Autodesk Fusion 360 part; units mm, degrees
sketch "Sketch1" plane through (0, 0, 0) normal (0, 1, 0) x (1, 0, 0)
  circle A0 centre (-14.1, 0) radius 1.6
  circle A1 centre (14.1, 0) radius 1.6
  line L0 (17.6, 1.5) -> (17.6, -11.5)
  line L1 (12.6, -16.5) -> (-12.6, -16.5)
  line L2 (-17.6, -11.5) -> (-17.6, 1.5)
  line L3 (10.6, 1.5) -> (10.6, -7.5)
  line L4 (-10.6, -7.5) -> (-10.6, 1.5)
  line L5 (12.6, 3.5) -> (15.6, 3.5)
  line L6 (-15.6, 3.5) -> (-12.6, 3.5)
  arc A2 (-17.6, -11.5) -> (-12.6, -16.5) centre (-12.6, -11.5) ccw
  arc A3 (12.6, -16.5) -> (17.6, -11.5) centre (12.6, -11.5) ccw
  arc A4 (-15.6, 3.5) -> (-17.6, 1.5) centre (-15.6, 1.5) ccw
  arc A5 (-10.6, 1.5) -> (-12.6, 3.5) centre (-12.6, 1.5) ccw
  arc A6 (12.6, 3.5) -> (10.6, 1.5) centre (12.6, 1.5) ccw
  arc A7 (17.6, 1.5) -> (15.6, 3.5) centre (15.6, 1.5) ccw
  line L7 (10.6, -7.5) -> (10.6, -9.5)
  line L8 (10.6, -9.5) -> (-10.6, -9.5)
  line L9 (-10.6, -9.5) -> (-10.6, -7.5)
  dimension "d2" = 14.1
  dimension "d3" = 3.2
  dimension "d4" = 3.2
  dimension "d11" = 5
  dimension "d12" = 2
extrude "Extrude1" add sketch "Sketch1" along normal blind 7.5
sketch "Sketch2" plane through (0, 0, 9.5) normal (0, 0, -1) x (1, 0, 0)
  line L0 (8.6, 0) -> (-8.6, 0)
  line L1 (-12.6, 0) -> (12.6, 0)
  line L2 (-8, 0) -> (-2.6967, 0) construction
  line L3 (-12.6, 0) -> (12.6, 0)
  line L4 (10.6, 0) -> (-10.6, 0)
  line L5 (-10.6, 0) -> (-10.6, -7.5)
  line L6 (-10.6, -7.5) -> (10.6, -7.5)
  line L7 (10.6, -7.5) -> (10.6, 0)
  circle A0 centre (8, -3.75) radius 1.6
  line L8 (-12.6, -7.5) -> (-12.6, 0)
  line L9 (8, 0) -> (4.25, -3.75)
  line L10 (12.6, -7.5) -> (-12.6, -7.5)
  line L11 (0, -3.75) -> (8, -3.75)
  circle A1 centre (-8, -3.75) radius 1.6
  line L12 (12.6, 0) -> (12.6, -7.5)
  line L13 (-8, 0) -> (-4.25, -3.75)
  line L14 (0, -3.75) -> (-8, -3.75)
  point P0 (0, -3.75)
extrude "Extrude2" cut sketch "Sketch2" against normal blind 8 contours A0 | A1 | L0 L1 L3 L4 L9 L11 L13 L14
fillet "Fillet2" radius 1 4 edges at (-8, 0, 13) (-4.25, 3.75, 13) (4.25, 3.75, 13) (8, 0, 13)
chamfer "Chamfer5" distance 0.5 angle 45 44 edges at (-10.6, 7.5, 4) (-11.1858, 7.5, -2.9142) (-14.1, 7.5, -3.5) (-17.0142, 7.5, -2.9142) (-17.6, 7.5, 5) (-16.1355, 7.5, 15.0355) (0, 7.5, 16.5) (16.1355, 7.5, 15.0355) (17.6, 7.5, 5) (17.0142, 7.5, -2.9142) (14.1, 7.5, -3.5) (11.1858, 7.5, -2.9142) (10.6, 7.5, 4) (0, 7.5, 9.5) (-10.6, 0, 4) (-11.1858, 0, -2.9142) (-14.1, 0, -3.5) (-17.0142, 0, -2.9142) (-17.6, 0, 5) (-16.1355, 0, 15.0355) (-10.5071, 0, 16.5) (-8.0315, 0.0761, 16.5) (-6.125, 1.875, 16.5) (-4.2185, 3.6739, 16.5) (0, 3.75, 16.5) (4.2185, 3.6739, 16.5) (6.125, 1.875, 16.5) (8.0315, 0.0761, 16.5) (10.5071, 0, 16.5) (16.1355, 0, 15.0355) (17.6, 0, 5) (17.0142, 0, -2.9142) (14.1, 0, -3.5) (11.1858, 0, -2.9142) (10.6, 0, 4) (9.5071, 0, 9.5) (8.0315, 0.0761, 9.5) (6.125, 1.875, 9.5) (4.2185, 3.6739, 9.5) (0, 3.75, 9.5) (-4.2185, 3.6739, 9.5) (-6.125, 1.875, 9.5) (-8.0315, 0.0761, 9.5) (-9.5071, 0, 9.5)
Can you work these out from the model? Positions are in its coordinate system, mm. A direction names the side the tool comes from. Give positions to 0.01 mm unless a question says otherwise; leave off trailing zeros. Order: outer loops, then holes, each group sorted by start corner. A loop starts at its lowest first (then second) coordinate and runs counter-clockwise, first axis right, second up. Notation, with made-up numbers: (-25, 72) - (20, 72) arc R35 cw to (20, 110) - close; hole circle Ø4 at (40, 41.5). An arc over 180 degrees is marked (long way). Use a Markdown table: item, result. Add a question column.
Q1. Please list where these lines run through material, in increasing order: line 1 along X through (y, z) = (5.5, 6.75); line 2 along X through (y, z) = (4.75, 13.5); line 3 along X through (y, z) = (7, 0.5).
Q2. If we section it at B-B on z = 0: Write out the boundary of the cut face in (x, y), plus the area to 3 significant figures.
Q3. On a 3-axis mill with a long thin cutter (end or side, diameter ignored), from which of +Z, -Z, +X, -X, +Y, -Y can I reach the whole of each face in a straight line? I mean faces 4 (the flat face through (-6.282, 2.076, 9.746)), 5 (the flat face through (0, 3.75, 13)), 6 (the flat face through (-10.6, 4, 4)), 7 (the conical face through (11.43, 7.36, -2.65)). Say none if no direction works.
Q4. I'm going to push flat-ended pins straight in: pin 1 (3.5 mm diameter, centred on x = 8, y = 3.75, fed in from +Z); pin 2 (3 mm diameter, centred on x = 4.5, y = 3, fed in from -Z); pin 3 (6.5 mm diameter, centred on x = 1.5, z = 14, fed in from -Y); pin 4 (4 mm diameter, centred on x = 9, y = 2.5, fed in from -Z). Where does each tip first touch, or does it pass through?
Q5. If we section it at C-C on y = 2.5: Count the separate pieces of the cut face and the enclosed holes in it, plus the area to 3 significant figures.
Q6. If we mould it in two halves opening along Z, with no side actions, what happens to faces 1 (the flat face through (6.282, 2.076, 9.746)), 2 (the flat face through (17.6, 4, 5)), 3 (the cylindrical face through (-12.574, 3.698, 0.481))? For each: released by +Z, released by -Z, zero draft, split by the parting line, or undercut.
Q7. If we section it at A-A on y = 1: Write out the boundary of the cut face in (x, z).
Q8. If we section it at D-D on z = 2.75: Write out the boundary of the cut face in (x, y), plus the area to 3 significant figures.
Answers follow:
| question | item | result |
|---|---|---|
| 1 | line 1 | x = -17.6 to -10.6, 10.6 to 17.6 |
| 1 | line 2 | x = -17.18 to -9.25, -6.75 to 6.75, 9.25 to 17.18 |
| 1 | line 3 | x = -17.6 to -15.62, -12.58 to -10.6, 10.6 to 12.58, 15.62 to 17.6 |
| 2 | outline | (-17.6, 0.5) - (-17.1, 0) - (-15.7, 0) - (-15.7, 7.5) - (-17.1, 7.5) - (-17.6, 7) - close; (-12.5, 0) - (-11.1, 0) - (-10.6, 0.5) - (-10.6, 7) - (-11.1, 7.5) - (-12.5, 7.5) - close; (10.6, 0.5) - (11.1, 0) - (12.5, 0) - (12.5, 7.5) - (11.1, 7.5) - (10.6, 7) - close; (15.7, 0) - (17.1, 0) - (17.6, 0.5) - (17.6, 7) - (17.1, 7.5) - (15.7, 7.5) - close |
| 2 | area | 56.0 mm^2 |
| 3 | face 4 | -Z, -Y |
| 3 | face 5 | +Z, -Z, -Y |
| 3 | face 6 | -Z, +Y, -Y |
| 3 | face 7 | -Z, +Y |
| 4 | pin 1 | stops at z = 16.5 |
| 4 | pin 2 | stops at z = 9.5 |
| 4 | pin 3 | stops at y = 3.25 |
| 4 | pin 4 | stops at z = -2.7 |
| 5 | separate pieces | 4 |
| 5 | enclosed holes | 2 |
| 5 | area | 292 mm^2 |
| 6 | face 1 | released by -Z |
| 6 | face 2 | zero draft |
| 6 | face 3 | undercut |
| 7 | outline | (-17.6, -1.5) arc R2 ccw to (-15.6, -3.5) - (-12.6, -3.5) arc R2 ccw to (-10.6, -1.5) - (-10.6, 9.5) - (-7.71, 9.5) - (-7, 10) - (-7, 16) - (-7.71, 16.5) - (-12.6, 16.5) arc R5 ccw to (-17.6, 11.5) - close; (7, 10) - (7.71, 9.5) - (10.6, 9.5) - (10.6, -1.5) arc R2 ccw to (12.6, -3.5) - (15.6, -3.5) arc R2 ccw to (17.6, -1.5) - (17.6, 11.5) arc R5 ccw to (12.6, 16.5) - (7.71, 16.5) - (7, 16) - close; hole circle Ø3.2 at (-14.1, 0); hole circle Ø3.2 at (14.1, 0) |
| 8 | outline | (-17.6, 0.5) - (-17.1, 0) - (-11.1, 0) - (-10.6, 0.5) - (-10.6, 7) - (-11.1, 7.5) - (-17.1, 7.5) - (-17.6, 7) - close; (10.6, 0.5) - (11.1, 0) - (17.1, 0) - (17.6, 0.5) - (17.6, 7) - (17.1, 7.5) - (11.1, 7.5) - (10.6, 7) - close |
| 8 | area | 104 mm^2 |
